from build123d import *

# Parameters (mm, degrees)
F0_R     = 53.5
F0_R_2   = 8.5
F1_DEPTH = 4
F2_W     = 20.5
F2_H     = 18
F2_R     = 8.5
F3_DEPTH = 1
F4_W     = 14
F4_H     = 2
F5_DEPTH = 25


# Not quite as in the source:
# - a feature names something its author has since deleted; it is built from what else it names


with BuildPart() as f1:
    # F0 (on Front) → F1 (new body)
    with BuildSketch(Plane.XZ):
        Circle(F0_R)
        with Locations((0, 30.2263684571)):
            Circle(F0_R_2, mode=Mode.SUBTRACT)
    extrude(amount=F1_DEPTH)

    # F2 (on face) → F3 (cut)
    with BuildSketch(Plane.XZ.offset(4)):
        with Locations((0, 30.2263684571)):
            Rectangle(F2_W, F2_H)
        with Locations((0, 30.2263684571)):
            Circle(F2_R, mode=Mode.SUBTRACT)
    extrude(amount=-F3_DEPTH, mode=Mode.SUBTRACT)

    # F4 (on face) → F5 (cut)
    with BuildSketch(Plane.XZ.offset(4)):
        with Locations((-24.5, 32)):
            Rectangle(F4_W, F4_H)
    extrude(amount=-F5_DEPTH, mode=Mode.SUBTRACT)


solid = f1.part
Source: CAD feature listing. Evaluate the final solid. Frame: model axes, mm. A direction names the side the tool comes from. Coordinates: 2 decimals unless noted, no trailing zeros. Loops run counter-clockwise (first coordinate to the right, second up) from the corner with the lowest first, then second, coordinate; pieces in that order, holes last. Notation, with made-up numbers: (70.5, 54.25) - (83.5, 54.25) arc R20 ccw to (83.5, 65.25) - close; hole circle Ø4 at (-6.75, 11). An arc over 180 degrees is marked (long way). Return JSON: item names as keys, results as strings.
Q1. Section A-A, the plane x = 0. Return loops of the section in (y, z).
Results:
{"outline": "(-4, -53.5) - (0, -53.5) - (0, 21.73) - (-3, 21.73) - (-3, 21.23) - (-4, 21.23) - close; (-4, 39.23) - (-3, 39.23) - (-3, 38.73) - (0, 38.73) - (0, 53.5) - (-4, 53.5) - close"}
Q2. Mould query, pull axis Z, two halves, no side actions, for faces 3 (the cylindrical face through (-11.598, -1.972, -52.228)), 4 (the flat face through (-1, -4, 1)), 5 (the flat face through (-25, -2, 31)), 6 (the flat face through (-25, -2, 33)). Classes: released by +Z, released by -Z, zero draft, split by the parting line, or undercut.
Results:
{"face 3": "split by the parting line", "face 4": "zero draft", "face 5": "undercut", "face 6": "undercut"}
Q3. Section B-B, the plane y = -1.5. Return loops of the section in (x, z), plus the area to 3 significant figures.
Results:
{"outline": "circle Ø107 at (0, 0); hole (-31.5, 31) - (-17.5, 31) - (-17.5, 33) - (-31.5, 33) - close; hole circle Ø17 at (0, 30.23)", "area": "8,740 mm2"}
Q4. Access query for faces 1 (the flat face through (-7, -3, 36)), 2 (the flat face through (-1, 0, 1)). Directions: +Z, -Z, +X, -X, +Y, -Y. A direction counts if a zero-diameter tool reaches every point of the face in a straight line with its end or side. Return the directions, or none.
Results:
{"face 1": "-Y", "face 2": "+Z, -Z, +X, -X, +Y"}
Q5. Section D-D, the plane x = 19. Return loops of the section in (y, z), plus the area to 3 significant figures.
Results:
{"outline": "(-4, -50.01) - (0, -50.01) - (0, 50.01) - (-4, 50.01) - close", "area": "400 mm2"}
Q6. Material intervals for line 1 along Z through (x, y) = (0, -2.2); line 2 along X through (y, z) = (-2.55, 32); line 3 along X through (y, z) = (-2.65, 34.5), sorted ascending.
Results:
{"line 1": "-53.5 to 21.73, 38.73 to 53.5", "line 2": "-42.87 to -31.5, -17.5 to -8.31, 8.31 to 42.87", "line 3": "-40.89 to -7.35, 7.35 to 40.89"}
Q7. Contact query for flat-ended pins moving along their axis: P1, Ø0.8, axis at x = 4, y = -3.5, coming from the +Z side; P2, Ø2, axis at y = -2, z = 32, coming from the -X side; P3, Ø0.8, axis at y = -3.5, z = 32, coming from the -X side. Output: stop coordinate, or through.
Results:
{"P1": "z = 53.38", "P2": "x = -43.6", "P3": "x = -43.17"}
Q8. Section C-C, the plane x = -27.5. Return loops of the section in (y, z), plus the area to 3 significant figures.
Results:
{"outline": "(-4, -45.89) - (0, -45.89) - (0, 31) - (-4, 31) - close; (-4, 33) - (0, 33) - (0, 45.89) - (-4, 45.89) - close", "area": "359 mm2"}
